Design review of the part built by this model. Coordinates are the model's own, in mm. A direction names the side the tool comes from. Coordinates: 2 decimals unless noted, no trailing zeros. Loops run counter-clockwise (first coordinate to the right, second up) from the corner with the lowest first, then second, coordinate; pieces in that order, holes last. Notation, with made-up numbers: M -7.75,85 L -3.75,85 A18 cw -3.75,96 Z; hole C 74.25,38.25 d5. An arc over 180 degrees is marked long. Write item = value, one per line. Start each with the question number.
```python
from build123d import *

# Parameters (mm, degrees)
SKETCH1_W           = 195
SKETCH1_H           = 50
BOSS_EXTRUDE1_DEPTH = 35
BOSS_EXTRUDE4_DEPTH = 35
CUT_EXTRUDE5_REACH  = 142.211
SKETCH11_R          = 1.75
SKETCH5_R           = 2.1
CUT_EXTRUDE6_DEPTH  = 6
CUT_EXTRUDE7_DEPTH  = 27
SKETCH12_R          = 3.45
CUT_EXTRUDE8_DEPTH  = 12


with BuildPart() as part:
    # Sketch1 → Boss-Extrude1 (new body)
    with BuildSketch(Plane(origin=(0, 0, 0), x_dir=(1, 0, 0), z_dir=(0, 1, 0))):
        Rectangle(SKETCH1_W, SKETCH1_H)
    extrude(amount=BOSS_EXTRUDE1_DEPTH)

    # Sketch8 → Boss-Extrude4 (add)
    with BuildSketch(Plane(origin=(0, 0, 0), x_dir=(1, 0, 0), z_dir=(0, 1, 0))):
        Polygon((55.952478692, -69), (55.952478692, -25), (39.452478692, -25), (39.452478692, -94.486788844), (97.5, -94.486788844), (97.5, -25), (81.452478692, -25), (81.452478692, -69), align=None)
    boss_extrude4 = extrude(amount=BOSS_EXTRUDE4_DEPTH)

    # Sketch11 → Cut-Extrude5 (cut, up to next)
    with BuildSketch(Plane(origin=(0, 0, 0), x_dir=(1, 0, 0), z_dir=(0, 1, 0)), mode=Mode.PRIVATE) as cut_extrude5_sk1:
        with Locations(Location((75.005806844, -0.5, 0), (0, 0, 270))):
            Circle(SKETCH11_R)
    cut_extrude5_tool1 = extrude(cut_extrude5_sk1.sketch, amount=CUT_EXTRUDE5_REACH, mode=Mode.PRIVATE) & part.part
    # Sketch11 → Cut-Extrude5 (cut, up to next)
    with BuildSketch(Plane(origin=(0, 0, 0), x_dir=(1, 0, 0), z_dir=(0, 1, 0)), mode=Mode.PRIVATE) as cut_extrude5_sk2:
        with Locations(Location((60.005806844, -0.5, 0), (0, 0, 270))):
            Circle(SKETCH11_R)
    cut_extrude5_tool2 = extrude(cut_extrude5_sk2.sketch, amount=CUT_EXTRUDE5_REACH, mode=Mode.PRIVATE) & part.part
    # Sketch11 → Cut-Extrude5 (cut, up to next)
    with BuildSketch(Plane(origin=(0, 0, 0), x_dir=(1, 0, 0), z_dir=(0, 1, 0)), mode=Mode.PRIVATE) as cut_extrude5_sk3:
        with Locations(Location((60.005806844, -10.5, 0), (0, 0, 270))):
            Circle(SKETCH11_R)
    cut_extrude5_tool3 = extrude(cut_extrude5_sk3.sketch, amount=CUT_EXTRUDE5_REACH, mode=Mode.PRIVATE) & part.part
    # Sketch11 → Cut-Extrude5 (cut, up to next)
    with BuildSketch(Plane(origin=(0, 0, 0), x_dir=(1, 0, 0), z_dir=(0, 1, 0)), mode=Mode.PRIVATE) as cut_extrude5_sk4:
        with Locations(Location((75.005806844, -10.5, 0), (0, 0, 270))):
            Circle(SKETCH11_R)
    cut_extrude5_tool4 = extrude(cut_extrude5_sk4.sketch, amount=CUT_EXTRUDE5_REACH, mode=Mode.PRIVATE) & part.part
    # Sketch11 → Cut-Extrude5 (cut, up to next)
    with BuildSketch(Plane(origin=(0, 0, 0), x_dir=(1, 0, 0), z_dir=(0, 1, 0)), mode=Mode.PRIVATE) as cut_extrude5_sk5:
        with Locations(Location((75.005806844, -79.986788844, 0), (0, 0, 270))):
            Circle(SKETCH11_R)
    cut_extrude5_tool5 = extrude(cut_extrude5_sk5.sketch, amount=CUT_EXTRUDE5_REACH, mode=Mode.PRIVATE) & part.part
    # Sketch11 → Cut-Extrude5 (cut, up to next)
    with BuildSketch(Plane(origin=(0, 0, 0), x_dir=(1, 0, 0), z_dir=(0, 1, 0)), mode=Mode.PRIVATE) as cut_extrude5_sk6:
        with Locations(Location((75.005806844, -89.986788844, 0), (0, 0, 270))):
            Circle(SKETCH11_R)
    cut_extrude5_tool6 = extrude(cut_extrude5_sk6.sketch, amount=CUT_EXTRUDE5_REACH, mode=Mode.PRIVATE) & part.part
    # Sketch11 → Cut-Extrude5 (cut, up to next)
    with BuildSketch(Plane(origin=(0, 0, 0), x_dir=(1, 0, 0), z_dir=(0, 1, 0)), mode=Mode.PRIVATE) as cut_extrude5_sk7:
        with Locations(Location((60.005806844, -79.986788844, 0), (0, 0, 270))):
            Circle(SKETCH11_R)
    cut_extrude5_tool7 = extrude(cut_extrude5_sk7.sketch, amount=CUT_EXTRUDE5_REACH, mode=Mode.PRIVATE) & part.part
    # Sketch11 → Cut-Extrude5 (cut, up to next)
    with BuildSketch(Plane(origin=(0, 0, 0), x_dir=(1, 0, 0), z_dir=(0, 1, 0)), mode=Mode.PRIVATE) as cut_extrude5_sk8:
        with Locations(Location((60.005806844, -89.986788844, 0), (0, 0, 270))):
            Circle(SKETCH11_R)
    cut_extrude5_tool8 = extrude(cut_extrude5_sk8.sketch, amount=CUT_EXTRUDE5_REACH, mode=Mode.PRIVATE) & part.part
    cut_extrude5_1 = cut_extrude5_tool1.solids().sort_by_distance((75.005807, 0, 0.5))[0]
    add(cut_extrude5_1, mode=Mode.SUBTRACT)
    cut_extrude5_2 = cut_extrude5_tool2.solids().sort_by_distance((60.005807, 0, 0.5))[0]
    add(cut_extrude5_2, mode=Mode.SUBTRACT)
    cut_extrude5_3 = cut_extrude5_tool3.solids().sort_by_distance((60.005807, 0, 10.5))[0]
    add(cut_extrude5_3, mode=Mode.SUBTRACT)
    cut_extrude5_4 = cut_extrude5_tool4.solids().sort_by_distance((75.005807, 0, 10.5))[0]
    add(cut_extrude5_4, mode=Mode.SUBTRACT)
    cut_extrude5_5 = cut_extrude5_tool5.solids().sort_by_distance((75.005807, 0, 79.986789))[0]
    add(cut_extrude5_5, mode=Mode.SUBTRACT)
    cut_extrude5_6 = cut_extrude5_tool6.solids().sort_by_distance((75.005807, 0, 89.986789))[0]
    add(cut_extrude5_6, mode=Mode.SUBTRACT)
    cut_extrude5_7 = cut_extrude5_tool7.solids().sort_by_distance((60.005807, 0, 79.986789))[0]
    add(cut_extrude5_7, mode=Mode.SUBTRACT)
    cut_extrude5_8 = cut_extrude5_tool8.solids().sort_by_distance((60.005807, 0, 89.986789))[0]
    add(cut_extrude5_8, mode=Mode.SUBTRACT)
    cut_extrude5 = cut_extrude5_1 + cut_extrude5_2 + cut_extrude5_3 + cut_extrude5_4 + cut_extrude5_5 + cut_extrude5_6 + cut_extrude5_7 + cut_extrude5_8  # Cut-Extrude5 as one shape, for the pattern or mirror that repeats it

    # Mirror2: Boss-Extrude4, Cut-Extrude5 across plane
    add(boss_extrude4.mirror(Plane(origin=(0, 0, 0), x_dir=(0, 0, 1), z_dir=(1, 0, 0))))
    add(cut_extrude5.mirror(Plane(origin=(0, 0, 0), x_dir=(0, 0, 1), z_dir=(1, 0, 0))), mode=Mode.SUBTRACT)

    # Sketch5 → Cut-Extrude6 (cut)
    with BuildSketch(Plane(origin=(0, 35, 0), x_dir=(1, 0, 0), z_dir=(0, 1, 0))):
        with Locations(Location((15, 14, 0), (0, 0, 270))):
            Circle(SKETCH5_R)
        with Locations(Location((-15, 14, 0), (0, 0, 270))):
            Circle(SKETCH5_R)
        with Locations(Location((-15, -6, 0), (0, 0, 270))):
            Circle(SKETCH5_R)
        with Locations(Location((15, -6, 0), (0, 0, 270))):
            Circle(SKETCH5_R)
    extrude(amount=-CUT_EXTRUDE6_DEPTH, mode=Mode.SUBTRACT)

    # Sketch15 → Cut-Extrude7 (cut)
    with BuildSketch(Plane(origin=(0, 35, 0), x_dir=(1, 0, 0), z_dir=(0, 1, 0))):
        Polygon((-29.2, 25), (-29.2, -1), (29.2, -1), (29.2, 25), (25.2, 25), (25.2, 21), (25.2, 3), (-25.2, 3), (-25.2, 21), (-25.2, 25), align=None)
    extrude(amount=-CUT_EXTRUDE7_DEPTH, mode=Mode.SUBTRACT)

    # Sketch12 → Cut-Extrude8 (cut)
    with BuildSketch(Plane.ZY.offset(-39.452478692)):
        with Locations((53.243394422, 30)):
            Circle(SKETCH12_R)
        with Locations((37.243394422, 30)):
            Circle(SKETCH12_R)
        with Locations((53.243394422, 5)):
            Circle(SKETCH12_R)
        with Locations((37.243394422, 5)):
            Circle(SKETCH12_R)
    cut_extrude8 = extrude(amount=-CUT_EXTRUDE8_DEPTH, mode=Mode.SUBTRACT)

    # Mirror3: Cut-Extrude8 across plane
    add(cut_extrude8.mirror(Plane(origin=(0, 0, 0), x_dir=(0, 0, 1), z_dir=(1, 0, 0))), mode=Mode.SUBTRACT)


solid = part.part
```
(1) To check wall thickness, follow L1, parallel to X at y = 22, z = -5; L2, parallel to Z at x = -75, y = 10; L3, parallel to X at y = 23.5, z = 35.5. State the ranges of each line that lie inside material, in increasing order.
(2) Take a section at B-B (z = -14). State the section outline as (x, y) points.
(3) Tool access review of faces 1 (the flat face through (2, 8, -2)), 2 (the flat face through (29.2, 22, -12)), 3 (the flat face through (-81.452, 17, 47)): name each direction out of +Z, -Z, +X, -X, +Y, -Y from which nothing blocks a thin tool from reaching the whole face with its end or side.
(4) Take a section at A-A (x = -15). State the section outline as (y, z) points, plus the area to 3 significant figures.
(5) Mouldability with a two-part tool opening along Z and no side actions: class faces 4 (the cylindrical face through (76.74, 17.26, 10.27)), 5 (the flat face through (-29.2, 22, -12)) as +Z half, -Z half, draft (parallel to the pull), parting line (faces both ways), or undercut.
(6) Insertion check: pin 1 (4 mm diameter, centred on x = -60.01, z = 89.99, fed in from -Y); pin 2 (6 mm diameter, centred on x = 72, z = 29.5, fed in from +Y). Each pin has a flat end and moves straight along its axis. Give the tip position at first contact, or say it passes through.
Results list:
q1.L1 = -97.5 to -29.2, -25.2 to 25.2, 29.2 to 97.5
q1.L2 = -25 to -1.25, 2.25 to 8.75, 12.25 to 25, 69 to 78.24, 81.74 to 88.24, 91.74 to 94.49
q1.L3 = -97.5 to -81.45, -55.95 to -39.45, 39.45 to 55.95, 81.45 to 97.5
q2.outline = M -97.5,0 L 97.5,0 L 97.5,35 L 29.2,35 L 29.2,8 L 25.2,8 L 25.2,35 L 17.1,35 L 17.1,29 L 12.9,29 L 12.9,35 L -12.9,35 L -12.9,29 L -17.1,29 L -17.1,35 L -25.2,35 L -25.2,8 L -29.2,8 L -29.2,35 L -97.5,35 Z
q3.face_1 = +Y
q3.face_2 = -Z, +Y
q3.face_3 = +Y, -Y
q4.outline = M 0,-25 L 35,-25 L 35,-16.1 L 29,-16.1 L 29,-11.9 L 35,-11.9 L 35,-3 L 8,-3 L 8,1 L 35,1 L 35,3.9 L 29,3.9 L 29,8.1 L 35,8.1 L 35,25 L 0,25 Z
q4.area = 1,590 mm^2
q5.face_4 = undercut
q5.face_5 = draft
q6.pin_1 = 0
q6.pin_2 = through
